Build history of the part. All positions in model axes, mm. Face numbers are marked on the shaded views. A direction names the side the tool comes from. Round coordinates to 2 decimals unless told otherwise and drop trailing zeros. Write each loop counter-clockwise with the first axis right and the second up, starting at its lowest first coordinate (ties: lowest second). Pieces come first, ordered by that corner, then holes. Notation, with made-up numbers: (-25, 78.5) - (27, 78.5) arc R8 ccw to (27, 88.5) - close; hole circle Ø1 at (49, 70). An arc over 180 degrees is marked (long way). Answer as a JSON object with one key per item and string values. Group by question number.
Item 1: Which spindle directions (+Z, -Z, +X, -X, +Y, -Y) get a long thin tool onto all of the face, cutting with end or side? Do the marked faces 1 and 2. Say none if no direction does.
Item 2: Slice it at D-D, the plane x = 7.25. List the corners of the cut face in (y, z).
Item 3: Two-plate mould, pull along Z, no slides. Class the marked faces 3, 4 and 5: +Z half, -Z half, draft (parallel to the pull), parting line (faces both ways), or undercut.
Item 4: Flat gauge pin, fed straight in: pin 1 (2 mm diameter, centred on y = -2.5, z = -18, fed in from +X). Where does the tip first touch, or does it go through?
Item 5: Slice it at C-C, the plane y = 0. List the corners of the cut face in (x, z).
Item 6: Slice it at A-A, the plane z = 0. List the corners of the cut face in (x, y), then the cut area to 3 significant figures.
Item 7: Slice it at B-B, the plane x = 24.25. List the corners of the cut face in (y, z), then the cut area to 3 significant figures.
Item 8: Probe line 1 (Y direction, x = 1.8, z = 0); line 2 (Z direction, x = 5.75, y = -1); line 3 (X direction, y = -24, z = -15). List the from-to ranges inside material, lowest first. Write a range as from..to.
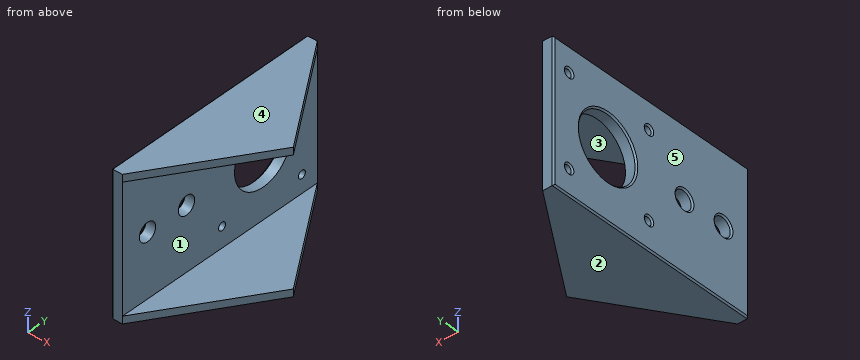
from build123d import *

# Parameters (mm, degrees)
SKETCH1_R           = 11.1125
SKETCH1_R_2         = 1.3589
SKETCH1_R_3         = 3.175
BOSS_EXTRUDE1_DEPTH = 3.81
BOSS_EXTRUDE2_DEPTH = 2.54
CHAMFER1_SIZE       = 0.5


with BuildPart() as part:
    # Sketch1 → Boss-Extrude1 (new body)
    with BuildSketch(Plane(origin=(0, 0, 0), x_dir=(0, 0, -1), z_dir=(1, 0, 0))):
        Polygon((21.79, -21.209), (21.79, -54.874917619), (-21.79, -54.874917619), (-21.79, -21.209), (-21.79, 21.209), (21.79, 21.209), align=None)
        with Locations(Location((0, 0, 0), (0, 0, 180))):
            Circle(SKETCH1_R, mode=Mode.SUBTRACT)
        with Locations(Location((15.588824177, 15.173169893, 0), (0, 0, 180))):
            Circle(SKETCH1_R_2, mode=Mode.SUBTRACT)
        with Locations(Location((-15.588824177, 15.173169893, 0), (0, 0, 180))):
            Circle(SKETCH1_R_2, mode=Mode.SUBTRACT)
        with Locations(Location((-14.746436813, -15.993096172, 0), (0, 0, 180))):
            Circle(SKETCH1_R_2, mode=Mode.SUBTRACT)
        with Locations(Location((14.746436813, -15.993096172, 0), (0, 0, 180))):
            Circle(SKETCH1_R_2, mode=Mode.SUBTRACT)
        with Locations(Location((0, -29.845, 0), (0, 0, 180))):
            Circle(SKETCH1_R_3, mode=Mode.SUBTRACT)
        with Locations(Location((0, -45.085, 0), (0, 0, 180))):
            Circle(SKETCH1_R_3, mode=Mode.SUBTRACT)
    extrude(amount=BOSS_EXTRUDE1_DEPTH)

    # Sketch15 → Boss-Extrude2 (add)
    with BuildSketch(Plane.XY.offset(21.79)):
        Polygon((3.81, 21.209), (29.21, -16.832958809), (3.81, -54.874917619), (0, -54.874917619), (0, 21.209), align=None)
    boss_extrude2 = extrude(amount=BOSS_EXTRUDE2_DEPTH)

    # Mirror1: Boss-Extrude2 across plane
    add(boss_extrude2.mirror(Plane.XY))

    # Chamfer1
    chamfer1_edges = [part.edges().sort_by_distance(p)[0] for p in [
        (0, 0, -11.1125),
        (0, 15.173169893, -16.947724177),
        (0, 15.173169893, 14.229924177),
        (0, -15.993096172, 13.387536813),
        (0, -15.993096172, -16.105336813),
        (0, -29.845, -3.175),
        (0, -45.085, -3.175),
        (0, -16.832958809, 24.33),
        (0, -16.832958809, -24.33),
        (0, -54.874917619, 0),
        (0, 21.209, 0),
    ]]
    chamfer(chamfer1_edges, length=CHAMFER1_SIZE)


solid = part.part
Geometry says:
{
 "1": {"face 1": "+X, +Y, -Y", "face 2": "-Z, +X, -X, +Y, -Y"},
 "2": {"outline": "(-49.72, -24.33) - (16.06, -24.33) - (16.06, -21.79) - (-49.72, -21.79) - close; (-49.72, 21.79) - (16.06, 21.79) - (16.06, 24.33) - (-49.72, 24.33) - close"},
 "3": {"face 3": "undercut", "face 4": "+Z half", "face 5": "draft"},
 "4": {"pin 1": "stops at x = 3.81"},
 "5": {"outline": "(0, -23.83) - (0.5, -24.33) - (17.97, -24.33) - (17.97, -21.79) - (3.81, -21.79) - (3.81, -11.11) - (0.5, -11.11) - (0, -11.61) - close; (0, 11.61) - (0.5, 11.11) - (3.81, 11.11) - (3.81, 21.79) - (17.97, 21.79) - (17.97, 24.33) - (0.5, 24.33) - (0, 23.83) - close"},
 "6": {"outline": "(0, -54.37) - (0.5, -54.87) - (3.81, -54.87) - (3.81, -48.26) - (0.5, -48.26) - (0, -48.76) - close; (0, -41.41) - (0.5, -41.91) - (3.81, -41.91) - (3.81, -33.02) - (0.5, -33.02) - (0, -33.52) - close; (0, -26.17) - (0.5, -26.67) - (3.81, -26.67) - (3.81, -11.11) - (0.5, -11.11) - (0, -11.61) - close; (0, 11.61) - (0.5, 11.11) - (3.81, 11.11) - (3.81, 21.21) - (0.5, 21.21) - (0, 20.71) - close", "area": "156 mm^2"},
 "7": {"outline": "(-24.26, -24.33) - (-9.4, -24.33) - (-9.4, -21.79) - (-24.26, -21.79) - close; (-24.26, 21.79) - (-9.4, 21.79) - (-9.4, 24.33) - (-24.26, 24.33) - close", "area": "75.5 mm^2"},
 "8": {"line 1": "y = -54.87..-48.26, -41.91..-33.02, -26.67..-11.11, 11.11..21.21", "line 2": "z = -24.33..-21.79, 21.79..24.33", "line 3": "x = 0..3.81"}
}
